Read the model definition and answer for the solid it produces. Units are mm, in the model's axes. Give positions to 0.01 mm unless a question says otherwise; leave off trailing zeros. Write each loop counter-clockwise with the first axis right and the second up, starting at its lowest first coordinate (ties: lowest second). Pieces come first, ordered by that corner, then holes. Notation, with made-up numbers: M -19.5,-11 L -1.5,-11 A12 cw -1.5,-3 Z; hole C 21.5,84 d2. An arc over 180 degrees is marked long. Answer as CSV lines item,"result". Start each with the question number.
```python
from build123d import *

# Parameters (mm, degrees)
SKETCH1_W           = 315.58
SKETCH1_H           = 3.175
BOSS_EXTRUDE1_DEPTH = 232.600000128
SKETCH5_W           = 3.175
SKETCH5_H           = 130.999992
CUT_EXTRUDE2_DEPTH  = 282.088108579
SKETCH7_R           = 3.302
CUT_EXTRUDE3_DEPTH  = 282.088108579
LPATTERN1_COUNT     = 3
LPATTERN1_PITCH     = 101.6


with BuildPart() as part:
    # Sketch1 → Boss-Extrude1 (new body)
    with BuildSketch(Plane.XY):
        Rectangle(SKETCH1_W, SKETCH1_H)
    extrude(amount=BOSS_EXTRUDE1_DEPTH)

    # Sketch5 → Cut-Extrude2 (cut, symmetric)
    with BuildSketch(Plane(origin=(0, 1.5875, 0), x_dir=(1, 0, 0), z_dir=(0, 1, 0))):
        with Locations((-156.2025, -65.499996)):
            Rectangle(SKETCH5_W, SKETCH5_H)
    cut_extrude2 = extrude(amount=CUT_EXTRUDE2_DEPTH, both=True, mode=Mode.SUBTRACT)

    # Mirror1: Cut-Extrude2 across plane
    add(cut_extrude2.mirror(Plane(origin=(0, 0, 0), x_dir=(0, 0, 1), z_dir=(1, 0, 0))), mode=Mode.SUBTRACT)

    # Sketch7 → Cut-Extrude3 (cut, through all)
    with BuildSketch(Plane.XZ.offset(1.5875)):
        with Locations(Location((107.495393219, 221.30835, 0), (0, 0, 270))):
            Circle(SKETCH7_R)
    cut_extrude3 = extrude(amount=-CUT_EXTRUDE3_DEPTH, mode=Mode.SUBTRACT)

    # LPattern1: Cut-Extrude3 ×3
    with Locations(*[(-i * LPATTERN1_PITCH, 0, 0) for i in range(1, LPATTERN1_COUNT)]):
        add(cut_extrude3, mode=Mode.SUBTRACT)


solid = part.part
```
1. Find section A-A on z = 118.5. Determine the outline of the cut face in (x, y) (1 decimal).
2. Given pin 1 (1 mm diameter, centred on y = 0.5, z = 64, fed in from -X) (3 decimals), flat-ended and moving along its own axis, determine where the tip first touches the part or whether it passes through.
3. Find the intervals of material crossed by line 1 (X direction, y = -1.05, z = 222); line 2 (X direction, y = 0.6, z = 223.5); line 3 (X direction, y = 0.95, z = 18) (3 decimals), in increasing order. Write a range as [from, to].
4. Determine the mould class of faces 1 (the face through (4.63, -0.02, 218.26)), 2 (the face through (-2, 1.588, 115)) for opening direction X: +X half, -X half, draft (parallel to the pull), parting line (faces both ways), or undercut.
Computed:
1,outline,"M -154.6,-1.6 L 154.6,-1.6 L 154.6,1.6 L -154.6,1.6 Z"
2,pin 1,"stops at x = -154.615"
3,line 1,"x = [-157.79, -98.93], [-92.48, 2.67], [9.12, 104.27], [110.72, 157.79]"
3,line 2,"x = [-157.79, -98.17], [-93.23, 3.43], [8.37, 105.03], [109.97, 157.79]"
3,line 3,"x = [-154.615, 154.615]"
4,face 1,"undercut"
4,face 2,"draft"
